Source: CAD feature listing. Evaluate the final solid. Frame: model axes, mm. Face numbers are marked on the shaded views. A direction names the side the tool comes from. Give positions to 0.01 mm unless a question says otherwise; leave off trailing zeros. Order: outer loops, then holes, each group sorted by start corner. A loop starts at its lowest first (then second) coordinate and runs counter-clockwise, first axis right, second up. Notation, with made-up numbers: M 48.25,-38.75 L 107.25,-38.75 A27 ccw 107.25,-13.75 Z; hole C 78.25,14.5 d10. An arc over 180 degrees is marked long. Return JSON: item names as keys, results as strings.
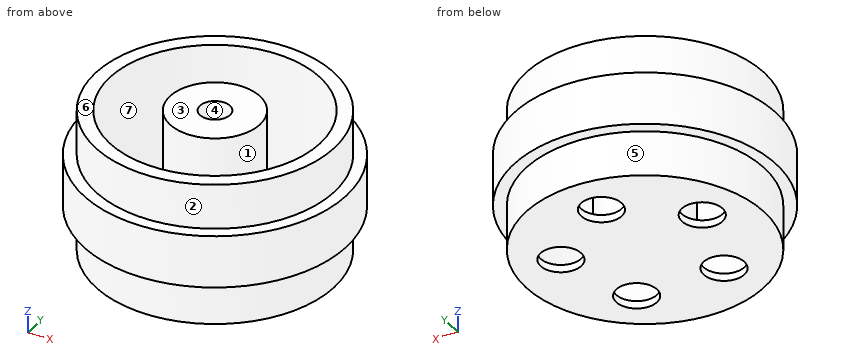
from build123d import *

# Parameters (mm, degrees)
F0_R      = 7.95
F1_DEPTH  = 3
F2_R      = 8.75
F3_DEPTH  = 3.5
F4_R      = 7.95
F5_DEPTH  = 3
F6_R      = 1.3579973099
F9_DEPTH  = 20.4
F8_R      = 7
F8_R_2    = 3
F8_R_3    = 1
F10_DEPTH = 9


with BuildPart() as f1:
    # F0 (on Top) → F1 (new body)
    with BuildSketch(Plane.XY):
        Circle(F0_R)
    extrude(amount=F1_DEPTH)

    # F2 (on face) → F3 (join)
    with BuildSketch(Plane.XY.offset(3)):
        Circle(F2_R)
    extrude(amount=F3_DEPTH)

    # F4 (on face) → F5 (join)
    with BuildSketch(Plane.XY.offset(6.5)):
        Circle(F4_R)
    extrude(amount=F5_DEPTH)

    # F6 (on face) → F9 (cut)
    with BuildSketch(Plane.XY.offset(9.5)):
        with Locations((0, 4.9537713639)):
            Circle(F6_R)
        with Locations((-4.7113165359, 1.5307995377)):
            Circle(F6_R)
        with Locations((-2.911753751, -4.0076852197)):
            Circle(F6_R)
        with Locations((2.911753751, -4.0076852197)):
            Circle(F6_R)
        with Locations((4.7113165359, 1.5307995377)):
            Circle(F6_R)
    extrude(amount=-F9_DEPTH, mode=Mode.SUBTRACT)

    # F8 (on face) → F10 (cut)
    with BuildSketch(Plane.XY.offset(9.5)):
        Circle(F8_R)
        Circle(F8_R_2, mode=Mode.SUBTRACT)
        Circle(F8_R_3)
    extrude(amount=-F10_DEPTH, mode=Mode.SUBTRACT)


solid = f1.part
1. Section query D-D (y = 4). Return loops of the section in (x, z), then the cut area to 3 significant figures.
Evaluation:
{"outline": "M -7.78,3 L -6.87,3 L -6.87,0 L -0.97,0 L -0.97,0.5 L -5.74,0.5 L -5.74,9.5 L -6.87,9.5 L -6.87,6.5 L -7.78,6.5 Z; M 0.97,0 L 6.87,0 L 6.87,3 L 7.78,3 L 7.78,6.5 L 6.87,6.5 L 6.87,9.5 L 5.74,9.5 L 5.74,0.5 L 0.97,0.5 Z", "area": "32.6 mm^2"}
2. Set-up query: the marked faces 5, 6 and 7. Return all of +Z, -Z, +X, -X, +Y, -Y with unobstructed straight access to the full face (end or side cutting, diameter ignored); none if empty.
Evaluation:
{"face 5": "-Z", "face 6": "+Z, +X, -X, +Y, -Y", "face 7": "+Z"}
3. Draft query along Y for the marked faces 1, 2, 3 and 4. Return one class per face: pulls with the +Y half, pulls with the -Y half, needs draft (parallel to the pull), parting line crosses it, or undercut.
Evaluation:
{"face 1": "undercut", "face 2": "parting line crosses it", "face 3": "needs draft", "face 4": "undercut"}
4. Ray query, probe 1 along Y at (x, z) = (2, 8.75); probe 2 along Z at (x, y) = (5, 3.5); probe 3 along Z at (x, y) = (7.75, -3.25). Return the intervals inside material, ascending.
Evaluation:
{"probe 1": "y = -7.69 to -6.71, -2.24 to 2.24, 6.71 to 7.69", "probe 2": "z = 0 to 0.5", "probe 3": "z = 3 to 6.5"}
5. Section query C-C (z = 5). Return loops of the section in (x, y), then the cut area to 3 significant figures.
Evaluation:
{"outline": "C 0,0 d17.5; C 0,0 d6; hole C 0,0 d14; hole C 0,0 d2", "area": "112 mm^2"}
6. First-contact query: pin 1 (1 mm diameter, centred on x = -5.5, z = 5, fed in from -Y); pin 2 (1 mm diameter, centred on y = 3, z = 5, fed in from -X); pin 3 (1 mm diameter, centred on y = -3.5, z = 1.5, fed in from +X). Flat tips, straight axial feed; report the tip coordinate or a pass-through.
Evaluation:
{"pin 1": "stops at y = -7.18", "pin 2": "stops at x = -8.39", "pin 3": "stops at x = 7.36"}
7. Section query A-A (x = 0). Return loops of the section in (y, z).
Evaluation:
{"outline": "M -8.75,3 L -7.95,3 L -7.95,0 L 3.6,0 L 3.6,0.5 L 3,0.5 L 3,9.5 L 1,9.5 L 1,0.5 L -1,0.5 L -1,9.5 L -3,9.5 L -3,0.5 L -7,0.5 L -7,9.5 L -7.95,9.5 L -7.95,6.5 L -8.75,6.5 Z; M 6.31,0 L 7.95,0 L 7.95,3 L 8.75,3 L 8.75,6.5 L 7.95,6.5 L 7.95,9.5 L 7,9.5 L 7,0.5 L 6.31,0.5 Z"}
8. Section query B-B (y = 2). Return loops of the section in (x, z).
Evaluation:
{"outline": "M -8.52,3 L -7.69,3 L -7.69,0 L -5.99,0 L -5.99,0.5 L -6.71,0.5 L -6.71,9.5 L -7.69,9.5 L -7.69,6.5 L -8.52,6.5 Z; M -3.44,0 L 3.44,0 L 3.44,0.5 L 2.24,0.5 L 2.24,9.5 L -2.24,9.5 L -2.24,0.5 L -3.44,0.5 Z; M 5.99,0 L 7.69,0 L 7.69,3 L 8.52,3 L 8.52,6.5 L 7.69,6.5 L 7.69,9.5 L 6.71,9.5 L 6.71,0.5 L 5.99,0.5 Z"}
